Design review of the part shown in the three views and the two pictorial views. Dimensions are in mm from the part's minimum x, y and z. A direction names the side the tool comes from. Give positions to 0.01 mm unless a question says otherwise; leave off trailing zeros. Loops run counter-clockwise (first coordinate to the right, second up) from the corner with the lowest first, then second, coordinate; pieces in that order, holes last.
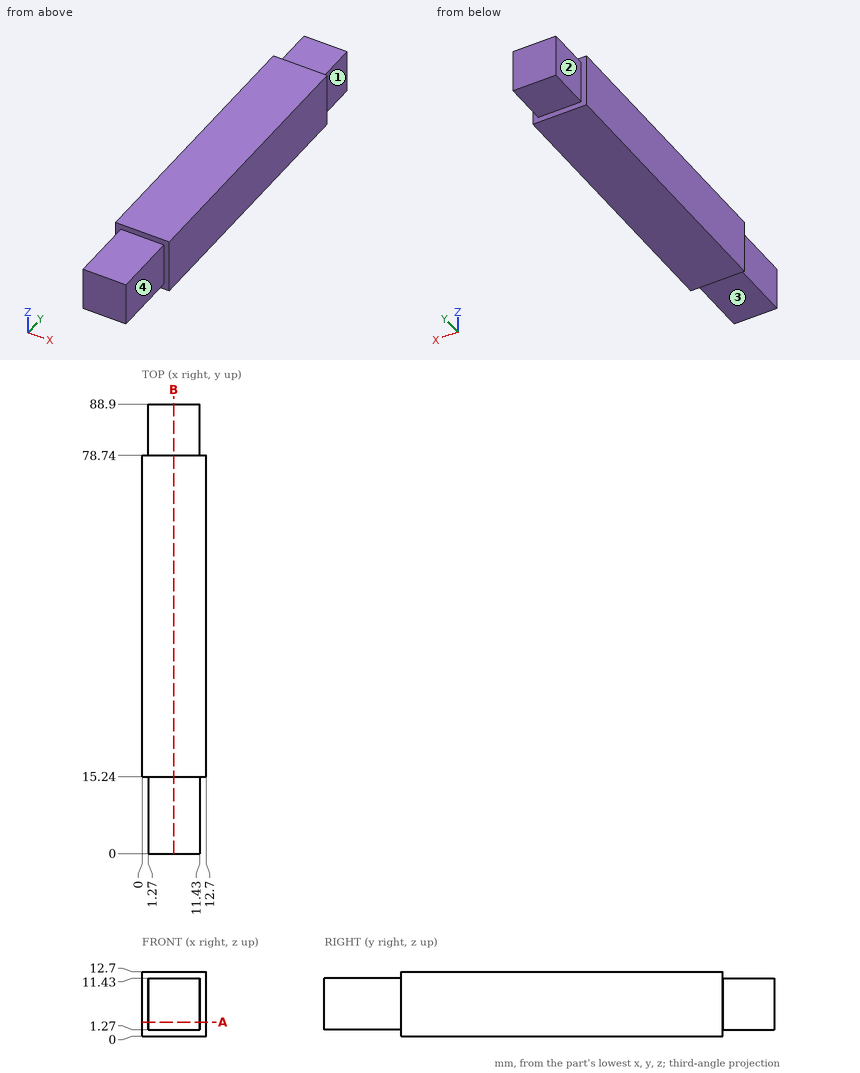
Q1. Consider section A-A on z = 2.75. Give the boundary of the cut face in (x, y), plus the area to 3 significant figures.
Answers:
outline: (0, 15.24) - (1.27, 15.24) - (1.27, 0) - (11.43, 0) - (11.43, 15.24) - (12.7, 15.24) - (12.7, 78.74) - (11.43, 78.74) - (11.43, 88.9) - (1.27, 88.9) - (1.27, 78.74) - (0, 78.74) - close
area: 1,060 mm2
Q2. Consider section B-B on x = 6.25. Give the boundary of the cut face in (y, z).
Answers:
outline: (0, 1.27) - (15.24, 1.27) - (15.24, 0) - (78.74, 0) - (78.74, 1.27) - (88.9, 1.27) - (88.9, 11.43) - (78.74, 11.43) - (78.74, 12.7) - (15.24, 12.7) - (15.24, 11.43) - (0, 11.43) - close
Q3. For pin 1 Ø5 at (x, y) = (6.5, 6) entering from -Z; pin 2 Ø5 at (x, y) = (5, 7.5) entering from +Z, all flat-tipped, find the tip position at first contact; note any pin that passes through.
Answers:
pin 1: stops at z = 1.27
pin 2: stops at z = 11.43
Q4. For probe 1 along Y at (x, z) = (8.5, 1); probe 2 along Z at (x, y) = (10, 7.5), list the stretches that pass through material, from the lowest coordinate up.
Answers:
probe 1: y = 15.24 to 78.74
probe 2: z = 1.27 to 11.43
Q5. Machinability: for the marked faces 1, 2, 3 and 4, which of the approach directions +Z, -Z, +X, -X, +Y, -Y give a long, thin tool a straight path to every point of the face, cutting with its end or side? Answer none if there is none.
Answers:
face 1: +Z, -Z, +X, +Y
face 2: +Z, -Z, -X, +Y
face 3: -Z, +X, -X, -Y
face 4: +Z, -Z, +X, -Y
